The model under review builds one solid part; all positions refer to its coordinate system, in mm. A direction names the side the tool comes from. Coordinates: 2 decimals unless noted, no trailing zeros. Order: outer loops, then holes, each group sorted by start corner. A loop starts at its lowest first (then second) coordinate and runs counter-clockwise, first axis right, second up. Notation, with made-up numbers: (64, -26.75) -> (108, -26.75) arc R16 cw to (108, -13.75) -> close; hole circle Ø10 at (10, 49). An arc over 180 degrees is marked (long way). Use CSV: the item, a comma, the result in double quotes. Start each with the question number.
```python
from build123d import *

# Parameters (mm, degrees)
F0_R     = 12.5
F1_DEPTH = 4
F2_R     = 15
F3_DEPTH = 75


with BuildPart() as f1:
    # F0 (on Front) → F1 (new body)
    with BuildSketch(Plane.XZ):
        Circle(F0_R)
    extrude(amount=F1_DEPTH)

    # F2 (on face) → F3 (join)
    with BuildSketch(Plane.XZ.offset(4)):
        Circle(F2_R)
    extrude(amount=F3_DEPTH)

    # F4: F1 across plane


with BuildPart() as f1_1:
    add(f1.part)
    add(f1.part.mirror(Plane.XZ))


solid = f1_1.part
```
Q1. Add section C-C, the plane z = 3.5. State the section outline as (x, y) points, then the cut area to 3 significant figures.
Q2. To check wall thickness, follow probe 1 along Y at (x, z) = (-10, 8.5); probe 2 along Z at (x, y) = (-0.75, 17.5); probe 3 along X at (y, z) = (70, 0.5). State the ranges of each line that lie inside material, in increasing order.
Q3. Add section B-B, the plane y = -42. State the section outline as (x, z) points.
Q4. Add section A-A, the plane x = -4.25. State the section outline as (y, z) points.
Q5. Draft analysis for pull direction Y (two halves, no side actions). For faces 3 (the flat face through (-3.4, -4, 12.3)), 4 (the flat face through (0, 79, 0)), 5 (the flat face through (0, -79, 0)), state which applies: +Y half, -Y half, draft (parallel to the pull), parting line (faces both ways), or undercut.
Q6. Clearance check with flat-ended pins moving along their axes: pin 1 Ø3 at (y, z) = (47.5, 4.5) entering from -X; pin 2 Ø8 at (y, z) = (15, -9) entering from -X; pin 3 Ø2 at (y, z) = (-32, 2) entering from -X. State where each tip first meets the part, or that it passes through.
Q7. For faces 1 (the cylindrical face through (-14.985, -40.975, 0.66)), 2 (the cylindrical face through (11.923, -0.056, 3.755)), list the 3-axis set-ups (+Z, -Z, +X, -X, +Y, -Y) from which the entire face can be reached by the end or side of a thin tool; tool diameter is ignored.
Answer block:
1,outline,"(-14.59, -79) -> (14.59, -79) -> (14.59, -4) -> (12, -4) -> (12, 4) -> (14.59, 4) -> (14.59, 79) -> (-14.59, 79) -> (-14.59, 4) -> (-12, 4) -> (-12, -4) -> (-14.59, -4) -> close"
1,area,"4,570 mm²"
2,probe 1,"y = -79 to -4, 4 to 79"
2,probe 2,"z = -14.98 to 14.98"
2,probe 3,"x = -14.99 to 14.99"
3,outline,"circle Ø30 at (0, 0)"
4,outline,"(-79, -14.39) -> (-4, -14.39) -> (-4, -11.76) -> (4, -11.76) -> (4, -14.39) -> (79, -14.39) -> (79, 14.39) -> (4, 14.39) -> (4, 11.76) -> (-4, 11.76) -> (-4, 14.39) -> (-79, 14.39) -> close"
5,face 3,"undercut"
5,face 4,"+Y half"
5,face 5,"-Y half"
6,pin 1,"stops at x = -14.7"
6,pin 2,"stops at x = -14.14"
6,pin 3,"stops at x = -14.97"
7,face 1,"+Y, -Y"
7,face 2,"none"
